Can you work these out from the model? Positions are in its coordinate system, mm. Face numbers are marked on the shaded views. A direction names the side the tool comes from. Give positions to 0.01 mm unless a question says otherwise; leave off trailing zeros. Order: outer loops, then holes, each group sorted by start corner. A loop starts at its lowest first (then second) coordinate and runs counter-clockwise, first axis right, second up. Notation, with made-up numbers: M -1.75,66.25 L 50.25,66.25 A25 ccw 50.25,100.25 Z; hole C 1,15 d6. An arc over 180 degrees is marked long. Write each question's results on one line, items separated by ' | '.
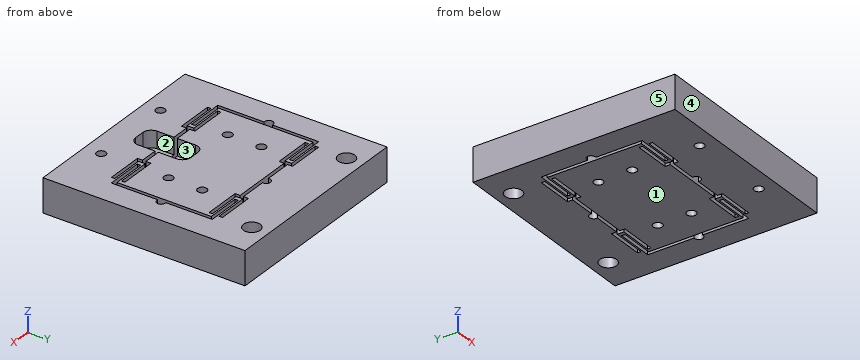
from build123d import *

# Parameters (mm, degrees)
SKETCH1_W                       = 76.2
SKETCH1_H                       = 76.2
BOSS_EXTRUDE1_DEPTH             = 6.35
CUT_EXTRUDE1_DEPTH              = 12.7
CUT_EXTRUDE2_DEPTH              = 12.7
F_1_4_0_25_DIAMETER_HOLE1_D     = 6.35
F_1_4_0_25_DIAMETER_HOLE1_DEPTH = 12.7
F_8_32_TAPPED_HOLE1_D           = 3.4544
F_8_32_TAPPED_HOLE1_DEPTH       = 12.7
SKETCH8_W                       = 10.16
SKETCH8_H                       = 20.828
CUT_EXTRUDE3_DEPTH              = 6.35
FILLET1_R                       = 3.175
FILLET2_R                       = 3.175
FILLET3_R                       = 3.175
FILLET4_R                       = 3.175
CUT_EXTRUDE6_REACH              = 14.7
SKETCH11_R                      = 1.5875


with BuildPart() as part:
    # Sketch1 → Boss-Extrude1 (new body, symmetric)
    with BuildSketch(Plane.XY):
        Rectangle(SKETCH1_W, SKETCH1_H)
    extrude(amount=BOSS_EXTRUDE1_DEPTH, both=True)

    # Sketch2 → Cut-Extrude1 (cut)
    with BuildSketch(Plane.XY.offset(6.35)):
        Polygon((14.605, 19.05), (28.575, 19.05), (28.575, -19.05), (14.605, -19.05), (14.605, -17.78), (27.305, -17.78), (27.305, 17.78), (14.605, 17.78), align=None)
    cut_extrude1 = extrude(amount=-CUT_EXTRUDE1_DEPTH, mode=Mode.SUBTRACT)

    # Mirror1: Cut-Extrude1 across plane
    add(cut_extrude1.mirror(Plane(origin=(0, 0, 0), x_dir=(0, 0, 1), z_dir=(1, 0, 0))), mode=Mode.SUBTRACT)

    # Sketch3 → Cut-Extrude2 (cut)
    with BuildSketch(Plane.XY.offset(6.35)):
        Polygon((25.781, 17.145), (25.781, 15.875), (11.811, 15.875), (11.811, 17.78), (-11.811, 17.78), (-11.811, 15.875), (-25.781, 15.875), (-25.781, 17.145), (-13.081, 17.145), (-13.081, 19.685), (-25.781, 19.685), (-25.781, 20.955), (-11.811, 20.955), (-11.811, 19.05), (11.811, 19.05), (11.811, 20.955), (25.781, 20.955), (25.781, 19.685), (13.081, 19.685), (13.081, 17.145), align=None)
    cut_extrude2 = extrude(amount=-CUT_EXTRUDE2_DEPTH, mode=Mode.SUBTRACT)

    # Mirror2: Cut-Extrude2 across plane
    add(cut_extrude2.mirror(Plane.ZX), mode=Mode.SUBTRACT)

    # 1/4 (0.25) Diameter Hole1
    with Locations(Plane.XY.offset(6.35)):
        with Locations((-25.4, 31.75), (25.4, 31.75)):
            Hole(F_1_4_0_25_DIAMETER_HOLE1_D / 2, depth=F_1_4_0_25_DIAMETER_HOLE1_DEPTH)

    # #8-32 Tapped Hole1
    with Locations(Plane.XY.offset(6.35)):
        with Locations((-15.875, 6.35), (15.875, 6.35), (15.875, -6.35), (-15.875, -6.35), (-15.875, -31.75), (15.875, -31.75)):
            Hole(F_8_32_TAPPED_HOLE1_D / 2, depth=F_8_32_TAPPED_HOLE1_DEPTH)

    # Sketch8 → Cut-Extrude3 (cut)
    with BuildSketch(Plane.XY.offset(6.35)):
        with Locations((0, -18.161)):
            Rectangle(SKETCH8_W, SKETCH8_H)
    extrude(amount=-CUT_EXTRUDE3_DEPTH, mode=Mode.SUBTRACT)

    # Fillet1
    fillet1_edges = [part.edges().sort_by_distance(p)[0] for p in [
        (-5.08, -7.747, 3.175),
    ]]
    fillet(fillet1_edges, radius=FILLET1_R)

    # Fillet2
    fillet2_edges = [part.edges().sort_by_distance(p)[0] for p in [
        (-5.08, -28.575, 3.175),
    ]]
    fillet(fillet2_edges, radius=FILLET2_R)

    # Fillet3
    fillet3_edges = [part.edges().sort_by_distance(p)[0] for p in [
        (5.08, -7.747, 3.175),
    ]]
    fillet(fillet3_edges, radius=FILLET3_R)

    # Fillet4
    fillet4_edges = [part.edges().sort_by_distance(p)[0] for p in [
        (5.08, -28.575, 3.175),
    ]]
    fillet(fillet4_edges, radius=FILLET4_R)

    # Sketch11 → Cut-Extrude6 (cut, up to next)
    with BuildSketch(Plane.XY.offset(6.35), mode=Mode.PRIVATE) as cut_extrude6_sk1:
        with Locations((0, 19.3675)):
            Circle(SKETCH11_R)
    cut_extrude6_tool1 = extrude(cut_extrude6_sk1.sketch, amount=-CUT_EXTRUDE6_REACH, mode=Mode.PRIVATE) & part.part
    add(cut_extrude6_tool1.solids().sort_by_distance((0, 19.3675, 6.35))[0], mode=Mode.SUBTRACT)
    # Sketch11 → Cut-Extrude6 (cut, up to next)
    with BuildSketch(Plane.XY.offset(6.35), mode=Mode.PRIVATE) as cut_extrude6_sk2:
        with Locations((28.8925, 0)):
            Circle(SKETCH11_R)
    cut_extrude6_tool2 = extrude(cut_extrude6_sk2.sketch, amount=-CUT_EXTRUDE6_REACH, mode=Mode.PRIVATE) & part.part
    add(cut_extrude6_tool2.solids().sort_by_distance((28.8925, 0, 6.35))[0], mode=Mode.SUBTRACT)
    # Sketch11 → Cut-Extrude6 (cut, up to next)
    with BuildSketch(Plane.XY.offset(6.35), mode=Mode.PRIVATE) as cut_extrude6_sk3:
        with Locations((0, -19.3675)):
            Circle(SKETCH11_R)
    cut_extrude6_tool3 = extrude(cut_extrude6_sk3.sketch, amount=-CUT_EXTRUDE6_REACH, mode=Mode.PRIVATE) & part.part
    add(cut_extrude6_tool3.solids().sort_by_distance((0, -19.3675, 6.35))[0], mode=Mode.SUBTRACT)
    # Sketch11 → Cut-Extrude6 (cut, up to next)
    with BuildSketch(Plane.XY.offset(6.35), mode=Mode.PRIVATE) as cut_extrude6_sk4:
        with Locations((-28.8925, 0)):
            Circle(SKETCH11_R)
    cut_extrude6_tool4 = extrude(cut_extrude6_sk4.sketch, amount=-CUT_EXTRUDE6_REACH, mode=Mode.PRIVATE) & part.part
    add(cut_extrude6_tool4.solids().sort_by_distance((-28.8925, 0, 6.35))[0], mode=Mode.SUBTRACT)


solid = part.part
(1) Imagine slicing it at B-B, the plane x = 21. Write out the boundary of the cut face in (y, z) (3 decimals).
Data:
outline: M -38.1,-6.35 L -20.955,-6.35 L -20.955,6.35 L -38.1,6.35 Z; M -19.685,-6.35 L -19.05,-6.35 L -19.05,6.35 L -19.685,6.35 Z; M -17.78,-6.35 L -17.145,-6.35 L -17.145,6.35 L -17.78,6.35 Z; M -15.875,-6.35 L 15.875,-6.35 L 15.875,6.35 L -15.875,6.35 Z; M 17.145,-6.35 L 17.78,-6.35 L 17.78,6.35 L 17.145,6.35 Z; M 19.05,-6.35 L 19.685,-6.35 L 19.685,6.35 L 19.05,6.35 Z; M 20.955,-6.35 L 38.1,-6.35 L 38.1,6.35 L 20.955,6.35 Z
(2) Imagine slicing it at A-A, the plane y = 3. Write out the boundary of the cut face in (x, z) (3 decimals), plus the area to 3 significant figures.
Data:
outline: M -38.1,-6.35 L -28.575,-6.35 L -28.575,6.35 L -38.1,6.35 Z; M -27.305,-6.35 L 27.305,-6.35 L 27.305,6.35 L -27.305,6.35 Z; M 28.575,-6.35 L 38.1,-6.35 L 38.1,6.35 L 28.575,6.35 Z | area: 935 mm2
(3) For the marked faces 1 and 2, which set-ups out of +Z, -Z, +X, -X, +Y, -Y let a thin tool reach every point of the face, with its end or its side?
Data:
face 1: -Z, +X, -X, +Y, -Y | face 2: +Z
(4) Imagine slicing it at C-C, the plane y = -6.35. Write out the boundary of the cut face in (x, z) (3 decimals), plus the area to 3 significant figures.
Data:
outline: M -38.1,-6.35 L -28.575,-6.35 L -28.575,6.35 L -38.1,6.35 Z; M -27.305,-6.35 L -17.602,-6.35 L -17.602,6.35 L -27.305,6.35 Z; M -14.148,-6.35 L 14.148,-6.35 L 14.148,6.35 L -14.148,6.35 Z; M 17.602,-6.35 L 27.305,-6.35 L 27.305,6.35 L 17.602,6.35 Z; M 28.575,-6.35 L 38.1,-6.35 L 38.1,6.35 L 28.575,6.35 Z | area: 848 mm2
(5) I need wall thicknesses on L1, parallel to X at y = -12.5, z = -1.75 (3 decimals); L2, parallel to X at y = 0, z = -1.75 (3 decimals); L3, parallel to Y at x = -6, z = -5. Which ranges of each line are inside material? Lowest first, please. Write a range as from..to.
Data:
L1: x = -38.1..-28.575, -27.305..27.305, 28.575..38.1 | L2: x = -38.1..-30.48, -27.305..27.305, 30.48..38.1 | L3: y = -38.1..-19.05, -17.78..17.78, 19.05..38.1
(6) We'd pull the mould along X, two halves only. Please class the marked faces 3, 4 and 5: +X half, -X half, draft (parallel to the pull), parting line (faces both ways), or undercut.
Data:
face 3: undercut | face 4: draft | face 5: -X half
(7) Will this pin go through, and if not, where does the flat tip stop? P1, Ø3, axis at x = -2, y = -21.5, coming from the +Z side.
Data:
P1: stops at z = 0
(8) Imagine slicing it at D-D, the plane x = 0. Write out the boundary of the cut face in (y, z) (3 decimals), plus the area to 3 significant figures.
Data:
outline: M -38.1,-6.35 L -20.955,-6.35 L -20.955,0 L -28.575,0 L -28.575,6.35 L -38.1,6.35 Z; M -17.78,-6.35 L 17.78,-6.35 L 17.78,6.35 L -7.747,6.35 L -7.747,0 L -17.78,0 Z; M 20.955,-6.35 L 38.1,-6.35 L 38.1,6.35 L 20.955,6.35 Z | area: 775 mm2
